```python
from build123d import *

# Parameters (mm, degrees)
BOSS_EXTRUDE1_DEPTH = 20


with BuildPart() as part:
    # Sketch1 → Boss-Extrude1 (new body)
    with BuildSketch(Plane.XY):
        with BuildLine():
            Line((35, -90.14), (35, 0))
            ThreePointArc((35, 0), (-0.97108607, 34.986525861), (-34.94611382, -1.941424451))
            Line((-34.94611382, -1.941424451), (-29.953811845, -91.804078101))
            ThreePointArc((-29.953811845, -91.804078101), (-20.616469836, -111.933603913), (0, -120.14))
            Line((0, -120.14), (15, -120.14))
            ThreePointArc((15, -120.14), (18.16227766, -119.626832981), (21, -118.14))
            ThreePointArc((21, -118.14), (31.304951685, -105.792475842), (35, -90.14))
        make_face()
        with BuildLine():
            Line((30, -90.14), (30, 0))
            ThreePointArc((30, 0), (-0.832359488, 29.988450738), (-29.953811845, -1.664078101))
            Line((-29.953811845, -1.664078101), (-24.961509871, -91.526731751))
            ThreePointArc((-24.961509871, -91.526731751), (-17.18039153, -108.301336594), (0, -115.14))
            Line((0, -115.14), (15, -115.14))
            ThreePointArc((15, -115.14), (16.58113883, -114.88341649), (18, -114.14))
            ThreePointArc((18, -114.14), (26.83281573, -103.556407865), (30, -90.14))
        make_face(mode=Mode.SUBTRACT)
    extrude(amount=BOSS_EXTRUDE1_DEPTH)


solid = part.part
```
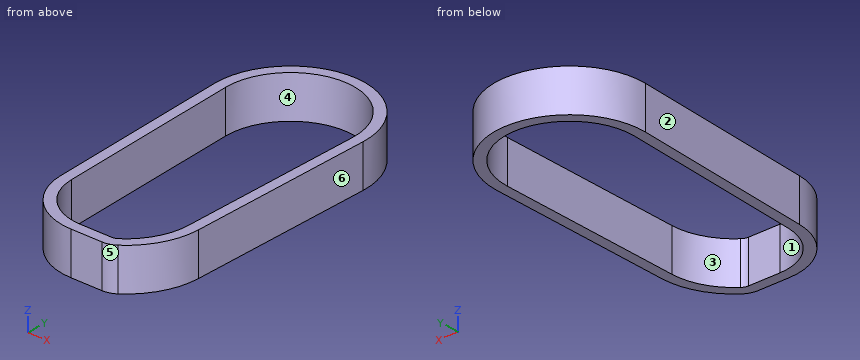
Can you work these out from the model? Positions are in its coordinate system, mm. Face numbers are marked on the shaded views. A direction names the side the tool comes from. Coordinates: 2 decimals unless noted, no trailing zeros. Loops run counter-clockwise (first coordinate to the right, second up) from the corner with the lowest first, then second, coordinate; pieces in that order, holes last. Notation, with made-up numbers: M 15,54.25 L 33,54.25 A24 ccw 33,83.25 Z; hole C -30,77 d7. An arc over 180 degrees is marked long. Put each result on its own line as item: value. Start each with the question number.
(1) I need wall thicknesses on probe 1 along X at (y, z) = (-1.5, 15.75); probe 2 along Y at (x, z) = (6, 1); probe 3 along Y at (x, z) = (-17.5, 5.5). Which ranges of each line are inside material? Lowest first, please.
(2) Which directions (+Z, -Z, +X, -X, +Y, -Y) give clear straight access to the entire face, cutting with the end or side of a thin tool? Please do the marked faces 1 and 2.
(3) We'd pull the mould along Y, two halves only. Please class the marked faces 3, 4, 5 and 6: +Y half, -Y half, draft (parallel to the pull), parting line (faces both ways), or undercut.
(4) Will these pins go through, and if not, where does the flat tip stop? pin 1 Ø2 at (x, z) = (5, 16) entering from +Y; pin 2 Ø7.5 at (x, z) = (11, 8.5) entering from +Y; pin 3 Ø12 at (x, z) = (24.5, 7) entering from +Y.
(5) Imagine slicing it at B-B on z = 7.25. List the corners of the cut face in (x, y) for me.
(6) Imagine slicing it at C-C on x = -15.5. List the corners of the cut face in (y, z) for me.
(7) Imagine slicing it at A-A on y = 5.5. List the corners of the cut face in (x, z) for me.
Worked answers:
1. probe 1: x = -34.97 to -29.96, 30 to 35
1. probe 2: y = -120.14 to -115.14, 29.39 to 34.48
1. probe 3: y = -114.51 to -107.99, 24.37 to 30.31
2. face 1: +Z, -Z
2. face 2: +Z, -Z, -X, -Y
3. face 3: undercut
3. face 4: undercut
3. face 5: -Y half
3. face 6: draft
4. pin 1: stops at y = 34.77
4. pin 2: stops at y = 34.24
4. pin 3: stops at y = 29.71
5. outline: M -34.95,-1.94 L -29.95,-91.8 A30 ccw 0,-120.14 L 15,-120.14 A10 ccw 21,-118.14 A35 ccw 35,-90.14 L 35,0 A35 ccw long Z; hole M -29.95,-1.66 L -24.96,-91.53 A25 ccw 0,-115.14 L 15,-115.14 A5 ccw 18,-114.14 A30 ccw 30,-90.14 L 30,0 A30 ccw long Z
6. outline: M -115.83,0 L -109.76,0 L -109.76,20 L -115.83,20 Z; M 25.69,0 L 31.38,0 L 31.38,20 L 25.69,20 Z
7. outline: M -34.57,0 L -29.49,0 L -29.49,20 L -34.57,20 Z; M 29.49,0 L 34.57,0 L 34.57,20 L 29.49,20 Z
